from build123d import *

# Parameters (mm, degrees)
SKETCH013_W     = 31.8
SKETCH013_H     = 31.8
SKETCH013_R     = 1.75
SKETCH013_W_2   = 29.000001
SKETCH013_H_2   = 2
PAD005_DEPTH    = 1
SKETCH014_W     = 31.8
SKETCH014_H     = 31.8
SKETCH014_W_2   = 29
SKETCH014_H_2   = 27.4
PAD006_DEPTH    = 32.4
SKETCH024_W     = 5.5
SKETCH024_H     = 27
POCKET010_DEPTH = 2


with BuildPart() as part:
    # Sketch013 (on Face2 of Binder003) → Pad005 (new body)
    with BuildSketch(Plane.XZ.offset(-33.95)):
        with Locations((13.749781, 0.8)):
            Rectangle(SKETCH013_W, SKETCH013_H)
        with Locations((5.24978, 9.3)):
            Circle(SKETCH013_R, mode=Mode.SUBTRACT)
        with Locations((22.24978, 9.3)):
            Circle(SKETCH013_R, mode=Mode.SUBTRACT)
        with Locations((22.24978, -7.7)):
            Circle(SKETCH013_R, mode=Mode.SUBTRACT)
        with Locations((5.24978, -7.7)):
            Circle(SKETCH013_R, mode=Mode.SUBTRACT)
        with Locations((13.74978, 0.8)):
            Rectangle(SKETCH013_W_2, SKETCH013_H_2, mode=Mode.SUBTRACT)
    extrude(amount=PAD005_DEPTH)

    # Sketch014 (on Face14 of Pad005) → Pad006 (join)
    with BuildSketch(Plane.XZ.offset(-32.95)):
        with Locations((13.74978, 0.8)):
            Rectangle(SKETCH014_W, SKETCH014_H)
        with Locations((13.74978, 0)):
            Rectangle(SKETCH014_W_2, SKETCH014_H_2, mode=Mode.SUBTRACT)
    extrude(amount=PAD006_DEPTH)

    # Sketch024 (on Face14 of Pad006) → Pocket010 (cut)
    with BuildSketch(Plane.XY.offset(16.7)):
        with Locations((13.74978, 14.05)):
            Rectangle(SKETCH024_W, SKETCH024_H)
    extrude(amount=-POCKET010_DEPTH, mode=Mode.SUBTRACT)


solid = part.part
Part model, mm, in its own coordinate system. A direction names the side the tool comes from. Coordinates: 2 decimals unless noted, no trailing zeros. Order: outer loops, then holes, each group sorted by start corner. A loop starts at its lowest first (then second) coordinate and runs counter-clockwise, first axis right, second up. Notation, with made-up numbers: (70, -24) - (118, -24) arc R32 ccw to (118, 14) - close; hole circle Ø8 at (21.5, 22). An arc over 180 degrees is marked (long way). Use CSV: the item, a comma, the result in double quotes.
Item 1: Saw through at A-A on x = 9.5. Give the cut face in (y, z).
Solved:
outline,"(0.55, -15.1) - (33.95, -15.1) - (33.95, -0.2) - (32.95, -0.2) - (32.95, -13.7) - (0.55, -13.7) - close; (0.55, 13.7) - (32.95, 13.7) - (32.95, 1.8) - (33.95, 1.8) - (33.95, 16.7) - (0.55, 16.7) - close"
Item 2: Saw through at C-C on z = -7.7. Give the number of separate pieces and of enclosed holes in the cut face, and give its area (3 significant figures).
Solved:
separate pieces,"3"
enclosed holes,"0"
area,"116 mm²"
Item 3: Saw through at B-B on y = 21.5. Give the cut face in (x, z).
Solved:
outline,"(-2.15, -15.1) - (29.65, -15.1) - (29.65, 16.7) - (16.5, 16.7) - (16.5, 14.7) - (11, 14.7) - (11, 16.7) - (-2.15, 16.7) - close; hole (-0.75, -13.7) - (28.25, -13.7) - (28.25, 13.7) - (-0.75, 13.7) - close"
Item 4: Mould opens along Z. For faces 6 (the face through (29.65, 33.5, 0.6)), 7 (the face through (28.25, 17, 0)), 8 (the face through (10, 17, 16.7)) say: +Z half, -Z half, draft (parallel to the pull), parting line (faces both ways), or undercut.
Solved:
face 6,"draft"
face 7,"undercut"
face 8,"+Z half"
Item 5: 3-axis set-ups, long thin cutter, end or side, ignore diameter. For faces 1 (the face through (-2.15, 17, 1)), 2 (the face through (29.65, 17, 1)), 3 (the face through (28.25, 33.5, 0.8)), 4 (the face through (11, 14, 16)), 5 (the face through (14, 17, -13.7)): which of +Z, -Z, +X, -X, +Y, -Y reach the whole face in a straight line?
Solved:
face 1,"+Z, -Z, -X, +Y, -Y"
face 2,"+Z, -Z, +X, +Y, -Y"
face 3,"+Y, -Y"
face 4,"+Z, -Y"
face 5,"-Y"
Item 6: Probe probe 1 along Z at (x, y) = (12, 7); probe 2 along X at (y, z) = (9.5, 0); probe 3 along X at (y, z) = (33, -7). List the from-to ranges inside material, lowest first.
Solved:
probe 1,"z = -15.1 to -13.7, 13.7 to 14.7"
probe 2,"x = -2.15 to -0.75, 28.25 to 29.65"
probe 3,"x = -2.15 to 3.65, 6.85 to 20.65, 23.85 to 29.65"
Item 7: Drop flat-ended pins along their axis: P1, Ø8, axis at x = 20, z = 12.5, coming from the -Y side; P2, Ø4.5, axis at x = 5.25, z = -7.7, coming from the -Y side; P3, Ø4.5, axis at x = 14, y = 15.5, coming from the +Z side. Give the stop position or say it passes through.
Solved:
P1,"stops at y = 0.55"
P2,"stops at y = 32.95"
P3,"stops at z = 14.7"
